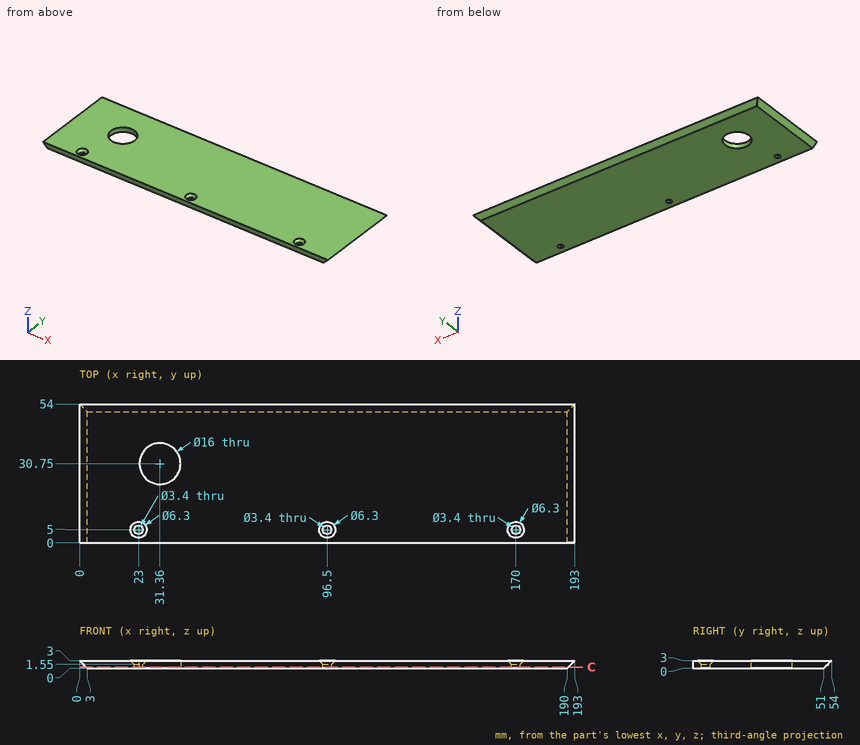
The figure shows three views and two pictorial views of one solid part (mm, origin at its lowest corner). Answer the questions. Give positions to 0.01 mm unless a question says otherwise; leave off trailing zeros. Order: outer loops, then holes, each group sorted by start corner. A loop starts at its lowest first (then second) coordinate and runs counter-clockwise, first axis right, second up. Notation, with made-up numbers: (46, 48.5) -> (50, 48.5) arc R24 ccw to (50, 63.5) -> close; hole circle Ø11 at (44.25, 27.5). An arc over 180 degrees is marked (long way). Answer as a JSON object with one key per item and string values. Group by question number.
Item 1: The part is cut by section C-C on z = 0.5. Write down the section's boundary in (x, y), and give its area (3 significant figures).
Item 2: Consider L1, parallel to X at y = 5, z = 0.85; L2, parallel to X at y = 5, z = 2.15; L3, parallel to Y at x = 96.5, z = 0.6. Determine where each line is inside the solid, lowest interval first. Write a range as from..to.
Item 3: A flat-ended cylindrical pin translates along its axis: pin 1 (1.5 mm diameter, centred on x = 154.5, z = 0.5, fed in from +Y). Find the tip coordinate at first contact, or state that the pin passes through.
Result set:
{
 "1": {"outline": "(2.5, 0) -> (190.5, 0) -> (190.5, 51.5) -> (2.5, 51.5) -> close; hole circle Ø3.4 at (23, 5); hole circle Ø16 at (31.36, 30.75); hole circle Ø3.4 at (96.5, 5); hole circle Ø3.4 at (170, 5)", "area": "9,450 mm²"},
 "2": {"L1": "2.15..21.3, 24.7..94.8, 98.2..168.3, 171.7..190.85", "L2": "0.85..20.7, 25.3..94.2, 98.8..167.7, 172.3..192.15", "L3": "0..3.3, 6.7..51.6"},
 "3": {"pin 1": "y = 52.25"}
}
